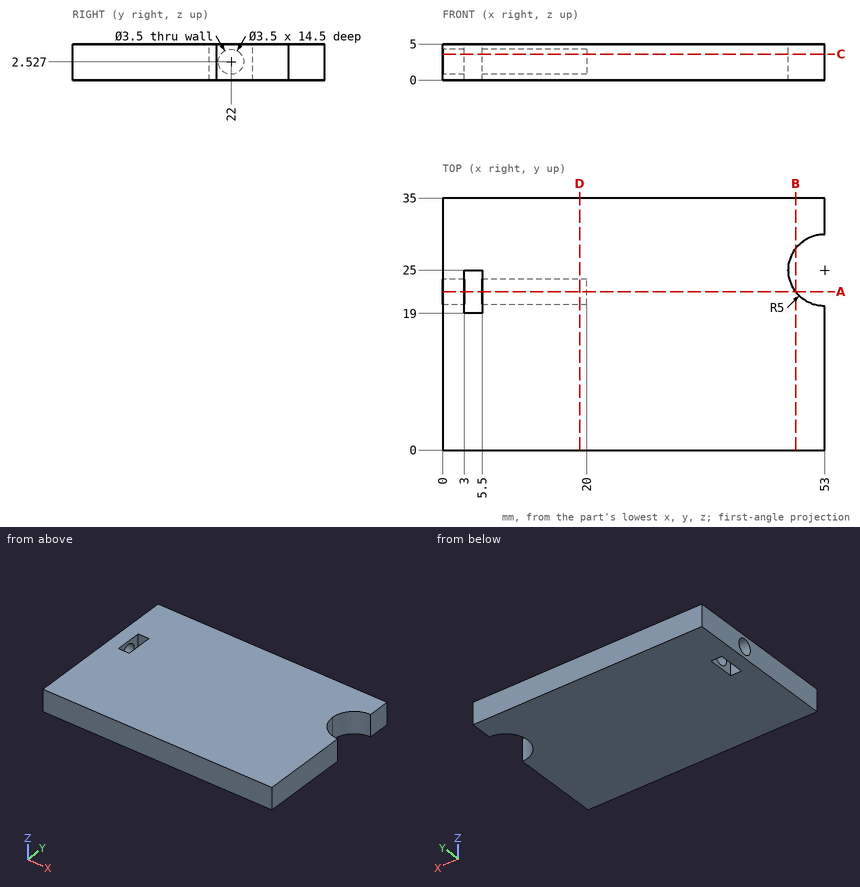
Check sheet for the drawn part. Datum: minimum x, y, z corner. Units: mm. Coordinates: 2 decimals unless noted, no trailing zeros. Loops run counter-clockwise (first coordinate to the right, second up) from the corner with the lowest first, then second, coordinate; pieces in that order, holes last. Notation, with made-up numbers: (-20.75, 53) - (26.25, 53) arc R16 cw to (26.25, 58) - close; hole circle Ø5 at (-8, -31). An arc over 180 degrees is marked (long way). Put each result on its own line as item: value.
Item 1: Scan lines: line 1 along Z through (x, y) = (1.65, 22); line 2 along Y through (x, z) = (9, 2.65) (1 decimal); line 3 along Y through (x, z) = (51, 1.5). Record each from-to range of solid material in increasing order.
Conclusion:
line 1: z = 0 to 0.78, 4.28 to 5
line 2: y = 0 to 20.3, 23.7 to 35
line 3: y = 0 to 20.42, 29.58 to 35
Item 2: Section check B-B (x = 49). Enter the section's corners in (y, z), then the cut area to 3 significant figures.
Conclusion:
outline: (0, 0) - (22, 0) - (22, 5) - (0, 5) - close; (28, 0) - (35, 0) - (35, 5) - (28, 5) - close
area: 145 mm2
Item 3: Section check D-D (x = 19). Enter the section's corners in (y, z).
Conclusion:
outline: (0, 0) - (35, 0) - (35, 5) - (0, 5) - close; hole circle Ø3.5 at (22, 2.53)
Item 4: Section check A-A (y = 22). Enter the section's corners in (x, z), then the cut area to 3 significant figures.
Conclusion:
outline: (0, 0) - (3, 0) - (3, 0.78) - (0, 0.78) - close; (0, 4.28) - (3, 4.28) - (3, 5) - (0, 5) - close; (5.5, 0) - (49, 0) - (49, 5) - (5.5, 5) - (5.5, 4.28) - (20, 4.28) - (20, 0.78) - (5.5, 0.78) - close
area: 171 mm2
Item 5: Gauge pin test, flat end, axial feed: pin 1 Ø2 at (y, z) = (22, 2.53) entering from +X. Record the tip position at first contact, or that the pin passes through.
Conclusion:
pin 1: stops at x = 50
Item 6: Section check C-C (z = 3.6). Enter the section's corners in (x, y), then the cut area to 3 significant figures.
Conclusion:
outline: (0, 0) - (53, 0) - (53, 20) arc R5 cw to (53, 30) - (53, 35) - (0, 35) - (0, 23.38) - (3, 23.38) - (3, 25) - (5.5, 25) - (5.5, 23.38) - (20, 23.38) - (20, 20.62) - (5.5, 20.62) - (5.5, 19) - (3, 19) - (3, 20.62) - (0, 20.62) - close
area: 1,750 mm2
